Input: part model. Units: mm. Frame: model coordinates. A direction names the side the tool comes from. Coordinates: 2 decimals unless noted, no trailing zeros. Order: outer loops, then holes, each group sorted by start corner. A loop starts at its lowest first (then second) coordinate and runs counter-clockwise, first axis right, second up. Notation, with made-up numbers: M -29,71 L 7,71 A24 cw 7,85 Z; hole C 55,24 d4. An arc over 180 degrees is marked long. One line per item, written item: value.
```python
from build123d import *

# Parameters (mm, degrees)
F0_R     = 2.54
F1_DEPTH = 25.4
F5_R     = 3.048
F6_DEPTH = 0.508
F4_R     = 3.048
F7_DEPTH = 0.508


with BuildPart() as f1:
    # F0 (on Top) → F1 (new body)
    with BuildSketch(Plane.XY):
        Circle(F0_R)
    extrude(amount=F1_DEPTH)

    # F5 (on offset) → F6 (join)
    with BuildSketch(Plane.XY.offset(23.622)):
        Circle(F5_R)
    extrude(amount=F6_DEPTH)

    # F4 (on offset) → F7 (join)
    with BuildSketch(Plane.XY.offset(1.778)):
        Circle(F4_R)
    extrude(amount=-F7_DEPTH)


solid = f1.part
```
(1) Cut plane A-A on y = 0. Output: boundary loops of the cut face in (x, z).
Data:
outline: M -3.05,1.27 L -2.54,1.27 L -2.54,0 L 2.54,0 L 2.54,1.27 L 3.05,1.27 L 3.05,1.78 L 2.54,1.78 L 2.54,23.62 L 3.05,23.62 L 3.05,24.13 L 2.54,24.13 L 2.54,25.4 L -2.54,25.4 L -2.54,24.13 L -3.05,24.13 L -3.05,23.62 L -2.54,23.62 L -2.54,1.78 L -3.05,1.78 Z
(2) Draft query along Z for faces 6 (the flat face through (-2, 2, 1.27)), 7 (the cylindrical face through (-0.33, 2.52, 24.76)), 8 (the flat face through (-2, 2, 23.622)). Return one class per face: released by +Z, released by -Z, zero draft, split by the parting line, or undercut.
Data:
face 6: released by -Z
face 7: zero draft
face 8: undercut
(3) First-contact query: pin 1 (1.5 mm diameter, centred on y = -1.5, z = 19, fed in from -X); pin 2 (2 mm diameter, centred on x = -2, y = -0.5, fed in from -Z); pin 3 (1 mm diameter, centred on y = 0, z = 12, fed in from -X); pin 4 (3 mm diameter, centred on x = 0.5, z = 21.5, fed in from +Y). Flat tips, straight axial feed; report the tip coordinate or a pass-through.
Data:
pin 1: stops at x = -2.43
pin 2: stops at z = 0
pin 3: stops at x = -2.54
pin 4: stops at y = 2.54
(4) Ray query, line 1 (Z direction, x = 2.75, y = -0.5); line 2 (X direction, y = 0, z = 13.5); line 3 (Y direction, x = 1, z = 22.25). Return the intervals inside material, ascending. Write a range as from..to.
Data:
line 1: z = 1.27..1.78, 23.62..24.13
line 2: x = -2.54..2.54
line 3: y = -2.33..2.33
(5) Cut plane C-C on z = 15.25. Output: boundary loops of the cut face in (x, y).
Data:
outline: C 0,0 d5.08
(6) Access query for faces 1 (the flat face through (-2, 2, 24.13)), 2 (the cylindrical face through (-0.4, 3.02, 1.53)), 3 (the cylindrical face through (-0.33, 2.52, 0.63)), 4 (the cylindrical face through (-0.33, 2.52, 12.55)), 5 (the flat face through (0, 0, 0)). Directions: +Z, -Z, +X, -X, +Y, -Y. A direction counts if a zero-diameter tool reaches every point of the face in a straight line with its end or side. Return the directions, or none.
Data:
face 1: +Z
face 2: +Z, -Z
face 3: -Z
face 4: none
face 5: -Z, +X, -X, +Y, -Y
